Check sheet for the modelled part. Datum: model origin and axes. Units: mm. A direction names the side the tool comes from. Round coordinates to 2 decimals unless told otherwise and drop trailing zeros. Loops run counter-clockwise (first coordinate to the right, second up) from the corner with the lowest first, then second, coordinate; pieces in that order, holes last. Notation, with made-up numbers: M -38.5,53.5 L -10.5,53.5 A15 ccw -10.5,57.5 Z; hole C 78.25,-38.75 d4. An arc over 180 degrees is marked long. Write item = value, one per line. Start each with the question number.
(1) Cross-section at B-B on y = -180. Record the boundary of the cut face in (x, z).
(2) Go/stop test with flat-tipped pins: P1, Ø6, axis at x = -1.5, z = 1.5, coming from the -Y side; P2, Ø1.2, axis at x = 4.25, y = -4.75, coming from the +Z side; P3, Ø4.5, axis at x = 3, y = -116, coming from the +Z side; P4, Ø1, axis at x = 1.5, z = 4.5, coming from the -Y side. Record where each tip stops, or that it passes through.
(3) Set-up check for faces 1 (the face through (10, -99, 0)), 2 (the face through (3.41, -151.73, -1.74)), 3 (the face through (-7, -101, 1)): record each of +Z, -Z, +X, -X, +Y, -Y from which the full face is reachable in a straight line by a thin tool's end or side.
(4) Cross-section at A-A on z = 1.5. Record the boundary of the cut face in (x, y), plus the area to 3 significant figures.
(5) Scan lines: L1, parallel to X at y = -116.95, z = -1.6; L2, parallel to X at y = -168, z = 1; L3, parallel to Y at x = 9.25, z = -3.25. Record each from-to range of solid material in increasing order. Write a range as from..to.
from build123d import *

# Parameters (mm, degrees)
PAD_DEPTH           = 200
SKETCH001_W         = 16
SKETCH001_H         = 199
POCKET_DEPTH        = 2
SKETCH002_W         = 14
SKETCH002_H         = 198
POCKET001_DEPTH     = 4
SKETCH003_W         = 16
SKETCH003_H         = 6
PAD001_DEPTH        = 2
SKETCH004_W         = 14
SKETCH004_H         = 2
POCKET002_DEPTH     = 4
POCKET003_DEPTH     = 1.5
SKETCH006_R         = 1
POCKET004_DEPTH     = 3
LINEARPATTERN_COUNT = 6
LINEARPATTERN_PITCH = 37.4


with BuildPart() as part:
    # Sketch → Pad (new body)
    with BuildSketch(Plane.XZ):
        with BuildLine():
            ThreePointArc((-9.233093, 5), (-9.658497, 4.11867), (-10, 3.201562))
            Line((-10, 3.201562), (-10, -3.201562))
            ThreePointArc((-10, -3.201562), (-9.658497, -4.11867), (-9.233093, -5))
            Line((-9.233093, -5), (9.233093, -5))
            ThreePointArc((9.233093, -5), (9.658497, -4.11867), (10, -3.201562))
            Line((10, 3.201562), (10, -3.201562))
            ThreePointArc((10, 3.201562), (9.658497, 4.11867), (9.233093, 5))
            Line((-9.233093, 5), (9.233093, 5))
        make_face()
    extrude(amount=PAD_DEPTH)

    # Sketch001 (on Face2 of Pad) → Pocket (cut)
    with BuildSketch(Plane(origin=(0, 0, 5), x_dir=(-1, 0, 0), z_dir=(0, 0, 1))):
        with Locations((0, 100.5)):
            Rectangle(SKETCH001_W, SKETCH001_H)
    extrude(amount=-POCKET_DEPTH, mode=Mode.SUBTRACT)

    # Sketch002 (on Face14 of Pocket) → Pocket001 (cut)
    with BuildSketch(Plane(origin=(0, 0, 3), x_dir=(-1, 0, 0), z_dir=(0, 0, 1))):
        with Locations((0, 101)):
            Rectangle(SKETCH002_W, SKETCH002_H)
    extrude(amount=-POCKET001_DEPTH, mode=Mode.SUBTRACT)

    # Sketch003 (on Face5 of Pocket001) → Pad001 (join)
    with BuildSketch(Plane.XZ.offset(200)):
        Rectangle(SKETCH003_W, SKETCH003_H)
    extrude(amount=PAD001_DEPTH)

    # Sketch004 (on Face18 of Pad001) → Pocket002 (cut)
    with BuildSketch(Plane(origin=(0, 0, 3), x_dir=(-1, 0, 0), z_dir=(0, 0, 1))):
        with Locations((0, 201)):
            Rectangle(SKETCH004_W, SKETCH004_H)
    extrude(amount=-POCKET002_DEPTH, mode=Mode.SUBTRACT)

    # Sketch005 (on Face27 of Pocket002) → Pocket003 (cut)
    with BuildSketch(Plane(origin=(0, 0, -1), x_dir=(-1, 0, 0), z_dir=(0, 0, 1))):
        with BuildLine():
            ThreePointArc((-5.85967, 6.979678), (-3.309445, 2.165845), (-4.450131, 7.492708))
            Line((-5.255331, 9.704978), (-4.450131, 7.492708))
            Line((-6.66487, 9.191948), (-5.255331, 9.704978))
            Line((-5.85967, 6.979678), (-6.66487, 9.191948))
        make_face()
        with BuildLine():
            ThreePointArc((4.450131, 7.492708), (3.309445, 2.165845), (5.85967, 6.979678))
            Line((6.66487, 9.191948), (5.85967, 6.979678))
            Line((5.255331, 9.704978), (6.66487, 9.191948))
            Line((4.450131, 7.492708), (5.255331, 9.704978))
        make_face()
    pocket003 = extrude(amount=-POCKET003_DEPTH, mode=Mode.SUBTRACT)

    # Sketch006 (on Face39 of Pocket003) → Pocket004 (cut)
    with BuildSketch(Plane(origin=(0, 0, -2.5), x_dir=(-1, 0, 0), z_dir=(0, 0, 1))):
        with Locations((-4.25, 4.75)):
            Circle(SKETCH006_R)
        with Locations((4.25, 4.75)):
            Circle(SKETCH006_R)
    pocket004 = extrude(amount=-POCKET004_DEPTH, mode=Mode.SUBTRACT)

    # LinearPattern: Pocket003, Pocket004 ×6
    with Locations(*[(0, -i * LINEARPATTERN_PITCH, 0) for i in range(1, LINEARPATTERN_COUNT)]):
        add(pocket003, mode=Mode.SUBTRACT)
        add(pocket004, mode=Mode.SUBTRACT)


solid = part.part
Result:
q1.outline = M -10,-3.2 A10.5 ccw -9.23,-5 L 9.23,-5 A10.5 ccw 10,-3.2 L 10,3.2 A10.5 ccw 9.23,5 L 8,5 L 8,3 L 7,3 L 7,-1 L -7,-1 L -7,3 L -8,3 L -8,5 L -9.23,5 A10.5 ccw -10,3.2 Z
q2.P1 = -202
q2.P2 = through
q2.P3 = -1
q2.P4 = -1
q3.face_1 = +Z, -Z, +X, +Y, -Y
q3.face_2 = +Z
q3.face_3 = +Z, -Y
q4.outline = M -10,-200 L -8,-200 L -8,-202 L -7,-202 L -7,-2 L 7,-2 L 7,-202 L 8,-202 L 8,-200 L 10,-200 L 10,0 L -10,0 Z
q4.area = 1,230 mm^2
q5.L1 = -10..-7, -1.5..1.5, 7..10
q5.L2 = -10..-7, 7..10
q5.L3 = -200..0
